```python
from build123d import *

# Parameters (mm, degrees)
F0_R     = 35.5
F0_R_2   = 6.25
F1_DEPTH = 1.2
F0_R_3   = 36.25
F2_DEPTH = 10
F3_R     = 1


with BuildPart() as f1:
    # F0 (on Top) → F1 (new body)
    with BuildSketch(Plane.XY):
        Circle(F0_R)
        with Locations((0, -21)):
            Circle(F0_R_2, mode=Mode.SUBTRACT)
        with Locations((-18.186533, 10.5)):
            Circle(F0_R_2, mode=Mode.SUBTRACT)
        Circle(F0_R_2, mode=Mode.SUBTRACT)
        with Locations((18.186533, 10.5)):
            Circle(F0_R_2, mode=Mode.SUBTRACT)
        with Locations((0, 21)):
            Circle(F0_R_2, mode=Mode.SUBTRACT)
    extrude(amount=-F1_DEPTH)

    # F0 (on Top) → F2 (join)
    with BuildSketch(Plane.XY):
        Circle(F0_R_3)
        Circle(F0_R, mode=Mode.SUBTRACT)
    extrude(amount=-F2_DEPTH)

    # F3
    f3_edges = [f1.edges().sort_by_distance(p)[0] for p in [
        (-36.25, 0, 0),
        (-35.5, 0, -1.2),
    ]]
    fillet(f3_edges, radius=F3_R)


solid = f1.part
```
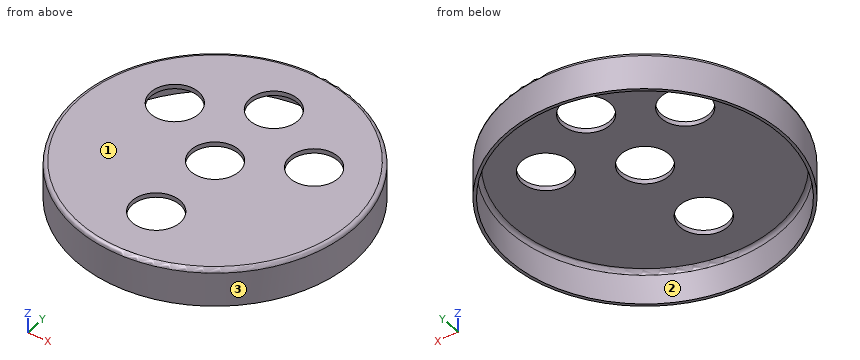
Read the model definition and answer for the solid it produces. Units are mm, in the model's axes. Face numbers are marked on the shaded views. Coordinates: 2 decimals unless noted, no trailing zeros. Write each loop counter-clockwise with the first axis right and the second up, starting at its lowest first coordinate (ties: lowest second). Pieces come first, ordered by that corner, then holes. Notation, with made-up numbers: (40.5, -29) - (84.5, -29) arc R15 cw to (84.5, -15) - close; hole circle Ø4 at (47.5, -30.75). An arc over 180 degrees is marked (long way). Answer as a JSON object with one key per item and string values. Group by question number.
1. A cutting plane is placed at D-D (y = 10.5). Give the number of separate pieces and of enclosed holes in the cut face, plus the area to 3 significant figures.
2. A cutting plane is placed at A-A (x = 0). Determine the outline of the cut face in (y, z).
3. Each of these flat-tipped pins is pushed along its axis until it touches: P1, Ø6, axis at y = -22.5, z = -4, coming from the -X side; P2, Ø10, axis at x = 12, y = -12.5, coming from the -Z side; P3, Ø3, axis at x = -22, z = -6, coming from the -Y side. Where does it stop, or does it pass through?
4. The mould has two halves that part along X. Classify the marked faces 1, 2 and 3: +X half, -X half, draft (parallel to the pull), parting line (faces both ways), or undercut.
5. Consider L1, parallel to Y at x = 0, z = -0.85; L2, parallel to Y at x = 0, z = -0.4; L3, parallel to Y at x = 0, z = -2.25. Determine where each line is inside the solid, lowest interval first. Write a range as [from, to].
6. A cutting plane is placed at B-B (y = 0). Determine the outline of the cut face in (x, z).
7. A cutting plane is placed at C-C (z = -8). Determine the outline of the cut face in (x, y), plus the area to 3 significant figures.
Worked out:
{
 "1": {"separate pieces": "3", "enclosed holes": "0", "area": "67.1 mm²"},
 "2": {"outline": "(-36.25, -10) - (-35.5, -10) - (-35.5, -2.2) arc R1 cw to (-34.5, -1.2) - (-27.25, -1.2) - (-27.25, 0) - (-35.25, 0) arc R1 ccw to (-36.25, -1) - close; (-14.75, -1.2) - (-6.25, -1.2) - (-6.25, 0) - (-14.75, 0) - close; (6.25, -1.2) - (14.75, -1.2) - (14.75, 0) - (6.25, 0) - close; (27.25, -1.2) - (34.5, -1.2) arc R1 cw to (35.5, -2.2) - (35.5, -10) - (36.25, -10) - (36.25, -1) arc R1 ccw to (35.25, 0) - (27.25, 0) - close"},
 "3": {"P1": "stops at x = -30.56", "P2": "stops at z = -1.2", "P3": "stops at y = -29.9"},
 "4": {"face 1": "draft", "face 2": "undercut", "face 3": "parting line"},
 "5": {"L1": "y = [-36.24, -27.25], [-14.75, -6.25], [6.25, 14.75], [27.25, 36.24]", "L2": "y = [-36.05, -27.25], [-14.75, -6.25], [6.25, 14.75], [27.25, 36.05]", "L3": "y = [-36.25, -35.5], [35.5, 36.25]"},
 "6": {"outline": "(-36.25, -10) - (-35.5, -10) - (-35.5, -2.2) arc R1 cw to (-34.5, -1.2) - (-6.25, -1.2) - (-6.25, 0) - (-35.25, 0) arc R1 ccw to (-36.25, -1) - close; (6.25, -1.2) - (34.5, -1.2) arc R1 cw to (35.5, -2.2) - (35.5, -10) - (36.25, -10) - (36.25, -1) arc R1 ccw to (35.25, 0) - (6.25, 0) - close"},
 "7": {"outline": "circle Ø72.5 at (0, 0); hole circle Ø71 at (0, 0)", "area": "169 mm²"}
}
